Part model, mm, in its own coordinate system. A direction names the side the tool comes from. Round coordinates to 2 decimals unless told otherwise and drop trailing zeros. Loops run counter-clockwise (first coordinate to the right, second up) from the corner with the lowest first, then second, coordinate; pieces in that order, holes last. Notation, with made-up numbers: M 29,-25 L 45,-25 A20 cw 45,11 Z; hole C 32.25,89.5 d7. An arc over 180 degrees is marked long. Put each result on its own line as item: value. Start each with the question number.
```python
from build123d import *

# Parameters (mm, degrees)
SALIENTE_EXTRUIR1_DEPTH = 12.7
CROQUIS2_R              = 2
CORTAR_EXTRUIR1_DEPTH   = 23
CROQUIS3_R              = 4
CORTAR_EXTRUIR2_DEPTH   = 5
CROQUIS4_R              = 3.96875
CORTAR_EXTRUIR3_DEPTH   = 15


with BuildPart() as part:
    # Croquis1 → Saliente-Extruir1 (new body)
    with BuildSketch(Plane.XY):
        with BuildLine():
            ThreePointArc((-9.971835338, -0.75), (10, 0), (-9.971835338, 0.75))
            Line((-9.971835338, 0.75), (-20, 0.75))
            Line((-20, 0.75), (-20, 15))
            Line((-20, 15), (20, 15))
            Line((20, 15), (20, -40))
            Line((20, -40), (-20, -40))
            Line((-20, -40), (-20, -0.75))
            Line((-20, -0.75), (-9.971835338, -0.75))
        make_face()
    extrude(amount=SALIENTE_EXTRUIR1_DEPTH)

    # Croquis2 → Cortar-Extruir1 (cut)
    with BuildSketch(Plane(origin=(0, 15, 0), x_dir=(1, 0, 0), z_dir=(0, 1, 0))):
        with Locations(Location((-15.000994664, -6.35, 0), (0, 0, 180))):
            Circle(CROQUIS2_R)
    extrude(amount=-CORTAR_EXTRUIR1_DEPTH, mode=Mode.SUBTRACT)

    # Croquis3 → Cortar-Extruir2 (cut)
    with BuildSketch(Plane(origin=(0, 15, 0), x_dir=(1, 0, 0), z_dir=(0, 1, 0))):
        with Locations(Location((-15.000994664, -6.35, 0), (0, 0, 180))):
            Circle(CROQUIS3_R)
    extrude(amount=-CORTAR_EXTRUIR2_DEPTH, mode=Mode.SUBTRACT)

    # Croquis4 → Cortar-Extruir3 (cut)
    with BuildSketch(Plane.XZ.offset(40)):
        with Locations(Location((-12.5, 6.35, 0), (0, 0, 270))):
            Circle(CROQUIS4_R)
        with Locations(Location((12.5, 6.35, 0), (0, 0, 270))):
            Circle(CROQUIS4_R)
    extrude(amount=-CORTAR_EXTRUIR3_DEPTH, mode=Mode.SUBTRACT)


solid = part.part
```
1. Mould opens along X. For faces 4 (the flat face through (-20, 8, 6)), 5 (the flat face through (13, -25, 6)), 6 (the cylindrical face through (16.435, -32.605, 6.867)), 7 (the flat face through (-12.8, -0.75, 6.3)) say: released by +X, released by -X, zero draft, split by the parting line, or undercut.
2. Cut at D-D, the plane z = 11. Give the cut face in (x, y).
3. Drop flat-ended pins along their axis: pin 1 (7 mm diameter, centred on x = 12.5, z = 6.35, fed in from -Y); pin 2 (4 mm diameter, centred on x = 13, y = -14.5, fed in from -Z); pin 3 (3 mm diameter, centred on x = -16, z = 7.5, fed in from +Y); pin 4 (8 mm diameter, centred on x = 1.5, y = 4, fed in from -Z). Give the stop position or say it passes through.
4. Cut at B-B, the plane z = 6.35. Give the cut face in (x, y).
5. Wall check: L1, parallel to Y at x = -13, z = 12.25; L2, parallel to X at y = -35.25, z = 6.35; L3, parallel to Y at x = 0, z = 4. Give the ranges that are in metal, low to high.
6. Cut at C-C, the plane x = -14. Give the cut face in (y, z), and give its area (3 significant figures).
7. Cut at A-A, the plane x = 0. Give the cut face in (y, z), and give its area (4 significant figures).
8. Which spindle directions (+Z, -Z, +X, -X, +Y, -Y) get a long thin tool onto all of the face, cutting with end or side? Do faces 1 (the cylindrical face through (-13, 5.4, 6.4)), 2 (the flat face through (-12.7, 0.75, 6.3)), 3 (the cylindrical face through (-9.818, -32.605, 9.275)). Say none if no direction does.
Results list:
1. face 4: released by -X
1. face 5: undercut
1. face 6: undercut
1. face 7: zero draft
2. outline: M -20,-40 L 20,-40 L 20,15 L -20,15 L -20,0.75 L -9.97,0.75 A10 cw long -9.97,-0.75 L -20,-0.75 Z
3. pin 1: stops at y = -25
3. pin 2: stops at z = 0
3. pin 3: stops at y = 10
3. pin 4: passes through
4. outline: M -20,-40 L -16.47,-40 L -16.47,-25 L -8.53,-25 L -8.53,-40 L 8.53,-40 L 8.53,-25 L 16.47,-25 L 16.47,-40 L 20,-40 L 20,15 L -11,15 L -11,10 L -13,10 L -13,0.75 L -9.97,0.75 A10 cw long -9.97,-0.75 L -13,-0.75 L -13,-8 L -17,-8 L -17,-0.75 L -20,-0.75 Z; M -20,0.75 L -17,0.75 L -17,10 L -19,10 L -19,15 L -20,15 Z
5. L1: y = -40 to -0.75, 0.75 to 15
5. L2: x = -20 to -16.47, -8.53 to 8.53, 16.47 to 20
5. L3: y = -40 to -10, 10 to 15
6. outline: M -40,0 L -0.75,0 L -0.75,4.62 L -8,4.62 L -8,8.08 L -0.75,8.08 L -0.75,12.7 L -40,12.7 L -40,10.02 L -25,10.02 L -25,2.68 L -40,2.68 Z; M 0.75,0 L 15,0 L 15,2.48 L 10,2.48 L 10,4.62 L 0.75,4.62 Z; M 0.75,8.08 L 10,8.08 L 10,10.22 L 15,10.22 L 15,12.7 L 0.75,12.7 Z
6. area: 473 mm^2
7. outline: M -40,0 L -10,0 L -10,12.7 L -40,12.7 Z; M 10,0 L 15,0 L 15,12.7 L 10,12.7 Z
7. area: 444.5 mm^2
8. face 1: +Y
8. face 2: +Z, -Z, -X
8. face 3: -Y
